```python
from build123d import *

# Parameters (mm, degrees)
F1_DEPTH = 50
F2_W     = 35
F2_H     = 50
F3_DEPTH = 25.5
F4_W     = 40
F4_H     = 50
F5_DEPTH = 35
F6_W     = 10
F6_H     = 40
F7_DEPTH = 25
F8_W     = 70
F8_H     = 75
F9_DEPTH = 20


with BuildPart() as f1:
    # F0 (on Front) → F1 (new body)
    with BuildSketch(Plane.XZ):
        Polygon((0, 75), (0, 0), (40.5, 0), (40.5, 50), (25, 50), (25, 75), align=None)
    extrude(amount=F1_DEPTH)

    # F2 (on face) → F3 (join)
    with BuildSketch(Plane.YZ.offset(40.5)):
        with Locations((-17.5, 25)):
            Rectangle(F2_W, F2_H)
    extrude(amount=F3_DEPTH)

    # F4 (on face) → F5 (join)
    with BuildSketch(Plane.YZ.offset(66)):
        with Locations((-20, 25)):
            Rectangle(F4_W, F4_H)
    extrude(amount=F5_DEPTH)

    # F6 (on face) → F7 (join)
    with BuildSketch(Plane.XY.offset(50)):
        with Locations((96, -20)):
            Rectangle(F6_W, F6_H)
    extrude(amount=F7_DEPTH)

    # F8 (on face) → F9 (join)
    with BuildSketch(Plane.YZ.offset(101)):
        with Locations((-35, 37.5)):
            Rectangle(F8_W, F8_H)
    extrude(amount=F9_DEPTH)


solid = f1.part
```
Check sheet for the modelled part. Datum: model origin and axes. Units: mm. A direction names the side the tool comes from. Coordinates: 2 decimals unless noted, no trailing zeros. Order: outer loops, then holes, each group sorted by start corner. A loop starts at its lowest first (then second) coordinate and runs counter-clockwise, first axis right, second up. Notation, with made-up numbers: (-26.75, 37.25) -> (-22.75, 37.25) arc R26 cw to (-22.75, 60.25) -> close; hole circle Ø2 at (67, 76). An arc over 180 degrees is marked (long way). Write each question's results on one line, items separated by ' | '. Start each with the question number.
1) Section check A-A (y = -48). Enter the section's corners in (x, z), and give its area (3 significant figures).
2) Draft check along X on faces 5 (the face through (60, 0, 29)), 6 (the face through (66, -38, 25)), 7 (the face through (91, -20, 62)), 8 (the face through (0, -25, 38)). Enter one of: pulls with the +X half, pulls with the -X half, needs draft (parallel to the pull), parting line crosses it, or undercut.
3) Section check C-C (y = -13.5). Enter the section's corners in (x, z).
4) Depth check by flat-ended pin: pin 1 (10.5 mm diameter, centred on x = 90, z = 38, fed in from -Y); pin 2 (5 mm diameter, centred on x = 88, y = -19.5, fed in from +Z); pin 3 (3 mm diameter, centred on x = 26, z = 60.5, fed in from -Y). Enter the tip coordinate at first touch or a pass-through.
5) Set-up check for faces 1 (the face through (20, -50, 38)), 2 (the face through (25, -25, 62)), 3 (the face through (101, -55, 38)), 4 (the face through (13, -25, 75)): record each of +Z, -Z, +X, -X, +Y, -Y from which the full face is reachable in a straight line by a thin tool's end or side.
6) Section check D-D (z = 28). Enter the section's corners in (x, y).
7) Section check B-B (z = 53.5). Enter the section's corners in (x, y).
8) Material ranges on line 1 along X through (y, z) = (-46, 35.5); line 2 along X through (y, z) = (-41.5, 65); line 3 along Y through (x, z) = (86, 25.5), recorded low to high.
Checked values:
1) outline: (0, 0) -> (40.5, 0) -> (40.5, 50) -> (25, 50) -> (25, 75) -> (0, 75) -> close; (101, 0) -> (121, 0) -> (121, 75) -> (101, 75) -> close | area: 4,150 mm²
2) face 5: needs draft | face 6: undercut | face 7: undercut | face 8: pulls with the -X half
3) outline: (0, 0) -> (121, 0) -> (121, 75) -> (91, 75) -> (91, 50) -> (25, 50) -> (25, 75) -> (0, 75) -> close
4) pin 1: y = -40 | pin 2: z = 50 | pin 3: y = -50
5) face 1: +Z, -Z, -X, -Y | face 2: +Z, +Y, -Y | face 3: +Z, -Z, -Y | face 4: +Z, +X, -X, +Y, -Y
6) outline: (0, -50) -> (40.5, -50) -> (40.5, -35) -> (66, -35) -> (66, -40) -> (101, -40) -> (101, -70) -> (121, -70) -> (121, 0) -> (0, 0) -> close
7) outline: (0, -50) -> (25, -50) -> (25, 0) -> (0, 0) -> close; (91, -40) -> (101, -40) -> (101, -70) -> (121, -70) -> (121, 0) -> (91, 0) -> close
8) line 1: 0 to 40.5, 101 to 121 | line 2: 0 to 25, 101 to 121 | line 3: -40 to 0
